```python
from build123d import *

# Parameters (mm, degrees)
EXTRUDE_1_OUTLINE_W = 110
EXTRUDE_1_OUTLINE_H = 90
EXTRUDE_1_DEPTH     = 3
SKETCH_2_R          = 1.5
CUT_EXTRUDE_1_DEPTH = 10
SKETCH_4_R          = 1
CUT_EXTRUDE_2_DEPTH = 10
SKETCH_5_W          = 10
SKETCH_5_H          = 54
CUT_EXTRUDE_3_DEPTH = 72.126647608
FILLET_1_R          = 3


# Read off the part's stored shape, not the designer's step: 凸台-拉伸1
with BuildPart() as part:
    # 凸台-拉伸1 outline → 凸台-拉伸1 (new body)
    with BuildSketch(Plane.XY):
        Rectangle(EXTRUDE_1_OUTLINE_W, EXTRUDE_1_OUTLINE_H)
    extrude(amount=EXTRUDE_1_DEPTH)

    # 草图2 → 切除-拉伸1 (cut)
    with BuildSketch(Plane.XY.offset(3)):
        with Locations((-47, 40)):
            Circle(SKETCH_2_R)
        with Locations((47, 30)):
            Circle(SKETCH_2_R)
        with Locations((47, -40)):
            Circle(SKETCH_2_R)
        with Locations((-47, -30)):
            Circle(SKETCH_2_R)
    extrude(amount=-CUT_EXTRUDE_1_DEPTH, mode=Mode.SUBTRACT)

    # 草图4 → 切除-拉伸2 (cut)
    with BuildSketch(Plane(origin=(0, 0, 0), x_dir=(-1, 0, 0), z_dir=(0, 0, -1))):
        with Locations((-7, 40)):
            Circle(SKETCH_4_R)
        with Locations((7, 40)):
            Circle(SKETCH_4_R)
        with Locations((-7, -40)):
            Circle(SKETCH_4_R)
        with Locations((7, -40)):
            Circle(SKETCH_4_R)
    extrude(amount=-CUT_EXTRUDE_2_DEPTH, mode=Mode.SUBTRACT)

    # 草图5 → 切除-拉伸3 (cut, through all)
    with BuildSketch(Plane.XY.offset(3)):
        with Locations((-18, 0)):
            Rectangle(SKETCH_5_W, SKETCH_5_H)
        Rectangle(SKETCH_5_W, SKETCH_5_H)
        with Locations((18, 0)):
            Rectangle(SKETCH_5_W, SKETCH_5_H)
    extrude(amount=-CUT_EXTRUDE_3_DEPTH, mode=Mode.SUBTRACT)

    # 圆角1
    fillet_1_edges = [part.edges().sort_by_distance(p)[0] for p in [
        (-23, -27, 1.5),
        (-23, 27, 1.5),
        (-13, 27, 1.5),
        (-13, -27, 1.5),
        (-5, -27, 1.5),
        (-5, 27, 1.5),
        (5, 27, 1.5),
        (5, -27, 1.5),
        (13, -27, 1.5),
        (13, 27, 1.5),
        (23, 27, 1.5),
        (23, -27, 1.5),
    ]]
    fillet(fillet_1_edges, radius=FILLET_1_R)


solid = part.part
```
Here's how the part is built. I have some questions about the finished solid (model axes, mm). Give positions to 0.01 mm unless a question says otherwise; leave off trailing zeros. Loops run counter-clockwise (first coordinate to the right, second up) from the corner with the lowest first, then second, coordinate; pieces in that order, holes last. Notation, with made-up numbers: M -20.75,75.25 L -11.75,75.25 A15 cw -11.75,92.25 Z; hole C 18.25,42 d11. An arc over 180 degrees is marked long. Use one line per item in the form item = value. Start each with the question number.
Q1. If we section it at B-B (y = 30): Write out the boundary of the cut face in (x, z).
Q2. Thinking about a two-plate mould opening in Y: for faces 1 (the flat face through (-55, -1, 1)), 2 (the flat face through (23, 0, 2)), 3 (the flat face through (-1, -45, 1)), which applies, +Y half, -Y half, draft (parallel to the pull), parting line (faces both ways), or undercut?
Q3. If we section it at C-C (z = 0.8): State how many separate pieces and enclosed holes the cut face has, then the cut area to 3 significant figures.
Q4. I need wall thicknesses on line 1 along Y through (x, z) = (47, 2.3); line 2 along Y through (x, z) = (7, 1.4); line 3 along X through (y, z) = (10.5, 0.35). Which ranges of each line are inside material? Lowest first, please.
Q5. If we section it at A-A (x = -47): Write out the boundary of the cut face in (y, z).
Q6. Will this pin go through, and if not, where does the flat tip stop? pin 1 Ø2.5 at (x, y) = (-7, -40) entering from +Z.
Taken from the geometry:
q1.outline = M -55,0 L 45.5,0 L 45.5,3 L -55,3 Z; M 48.5,0 L 55,0 L 55,3 L 48.5,3 Z
q2.face_1 = draft
q2.face_2 = undercut
q2.face_3 = -Y half
q3.separate_pieces = 1
q3.enclosed_holes = 11
q3.area = 8,260 mm^2
q4.line_1 = -45 to -41.5, -38.5 to 28.5, 31.5 to 45
q4.line_2 = -45 to -41, -39 to 39, 41 to 45
q4.line_3 = -55 to -23, -13 to -5, 5 to 13, 23 to 55
q5.outline = M -45,0 L -31.5,0 L -31.5,3 L -45,3 Z; M -28.5,0 L 38.5,0 L 38.5,3 L -28.5,3 Z; M 41.5,0 L 45,0 L 45,3 L 41.5,3 Z
q6.pin_1 = 3
